Part model, mm, in its own coordinate system. A direction names the side the tool comes from. Give positions to 0.01 mm unless a question says otherwise; leave off trailing zeros. Order: outer loops, then holes, each group sorted by start corner. A loop starts at its lowest first (then second) coordinate and runs counter-clockwise, first axis right, second up.
from build123d import *

# Parameters (mm, degrees)
BOSS_EXTRUDE1_DEPTH = 3
CUT_EXTRUDE1_DEPTH  = 54.310411741


with BuildPart() as part:
    # Sketch1 → Boss-Extrude1 (new body)
    with BuildSketch(Plane.XY):
        Polygon((0, 0), (0, 45), (5, 45), (5, 48), (15, 48), (15, 45), (23, 45), (23, 27.5), (20, 27.5), (20, 17.5), (23, 17.5), (23, 0), (15, 0), (15, -6), (5, -6), (5, 0), align=None)
    extrude(amount=BOSS_EXTRUDE1_DEPTH)

    # Sketch2 → Cut-Extrude1 (cut, through all)
    with BuildSketch(Plane.XY.offset(3)):
        with BuildLine():
            Line((2.1, 42), (5.9, 42))
            ThreePointArc((5.9, 42), (5.970710678, 41.970710678), (6, 41.9))
            Line((6, 41.9), (6, 39.4))
            ThreePointArc((6, 39.4), (5.970710678, 39.329289322), (5.9, 39.3))
            Line((5.9, 39.3), (2.1, 39.3))
            ThreePointArc((2.1, 39.3), (2.029289322, 39.329289322), (2, 39.4))
            Line((2, 39.4), (2, 41.9))
            ThreePointArc((2, 41.9), (2.029289322, 41.970710678), (2.1, 42))
        make_face()
        with BuildLine():
            Line((8.1, 42), (11.9, 42))
            ThreePointArc((11.9, 42), (11.970710678, 41.970710678), (12, 41.9))
            Line((12, 41.9), (12, 39.4))
            ThreePointArc((12, 39.4), (11.970710678, 39.329289322), (11.9, 39.3))
            Line((11.9, 39.3), (8.1, 39.3))
            ThreePointArc((8.1, 39.3), (8.029289322, 39.329289322), (8, 39.4))
            Line((8, 39.4), (8, 41.9))
            ThreePointArc((8, 41.9), (8.029289322, 41.970710678), (8.1, 42))
        make_face()
        with BuildLine():
            Line((14.1, 42), (17.9, 42))
            ThreePointArc((17.9, 42), (17.970710678, 41.970710678), (18, 41.9))
            Line((18, 41.9), (18, 39.4))
            ThreePointArc((18, 39.4), (17.970710678, 39.329289322), (17.9, 39.3))
            Line((17.9, 39.3), (14.1, 39.3))
            ThreePointArc((14.1, 39.3), (14.029289322, 39.329289322), (14, 39.4))
            Line((14, 39.4), (14, 41.9))
            ThreePointArc((14, 41.9), (14.029289322, 41.970710678), (14.1, 42))
        make_face()
        with BuildLine():
            Line((8.1, 37), (11.9, 37))
            ThreePointArc((11.9, 37), (11.970710678, 36.970710678), (12, 36.9))
            Line((12, 36.9), (12, 34.4))
            ThreePointArc((12, 34.4), (11.970710678, 34.329289322), (11.9, 34.3))
            Line((11.9, 34.3), (8.1, 34.3))
            ThreePointArc((8.1, 34.3), (8.029289322, 34.329289322), (8, 34.4))
            Line((8, 34.4), (8, 36.9))
            ThreePointArc((8, 36.9), (8.029289322, 36.970710678), (8.1, 37))
        make_face()
        with BuildLine():
            Line((14.1, 37), (17.9, 37))
            ThreePointArc((17.9, 37), (17.970710678, 36.970710678), (18, 36.9))
            Line((18, 36.9), (18, 34.4))
            ThreePointArc((18, 34.4), (17.970710678, 34.329289322), (17.9, 34.3))
            Line((17.9, 34.3), (14.1, 34.3))
            ThreePointArc((14.1, 34.3), (14.029289322, 34.329289322), (14, 34.4))
            Line((14, 34.4), (14, 36.9))
            ThreePointArc((14, 36.9), (14.029289322, 36.970710678), (14.1, 37))
        make_face()
        with BuildLine():
            Line((8.1, 32), (11.9, 32))
            ThreePointArc((11.9, 32), (11.970710678, 31.970710678), (12, 31.9))
            Line((12, 31.9), (12, 29.4))
            ThreePointArc((12, 29.4), (11.970710678, 29.329289322), (11.9, 29.3))
            Line((11.9, 29.3), (8.1, 29.3))
            ThreePointArc((8.1, 29.3), (8.029289322, 29.329289322), (8, 29.4))
            Line((8, 29.4), (8, 31.9))
            ThreePointArc((8, 31.9), (8.029289322, 31.970710678), (8.1, 32))
        make_face()
        with BuildLine():
            Line((14.1, 32), (17.9, 32))
            ThreePointArc((17.9, 32), (17.970710678, 31.970710678), (18, 31.9))
            Line((18, 31.9), (18, 29.4))
            ThreePointArc((18, 29.4), (17.970710678, 29.329289322), (17.9, 29.3))
            Line((17.9, 29.3), (14.1, 29.3))
            ThreePointArc((14.1, 29.3), (14.029289322, 29.329289322), (14, 29.4))
            Line((14, 29.4), (14, 31.9))
            ThreePointArc((14, 31.9), (14.029289322, 31.970710678), (14.1, 32))
        make_face()
        with BuildLine():
            Line((2.1, 37), (5.9, 37))
            ThreePointArc((5.9, 37), (5.970710678, 36.970710678), (6, 36.9))
            Line((6, 36.9), (6, 34.4))
            ThreePointArc((6, 34.4), (5.970710678, 34.329289322), (5.9, 34.3))
            Line((5.9, 34.3), (2.1, 34.3))
            ThreePointArc((2.1, 34.3), (2.029289322, 34.329289322), (2, 34.4))
            Line((2, 34.4), (2, 36.9))
            ThreePointArc((2, 36.9), (2.029289322, 36.970710678), (2.1, 37))
        make_face()
        with BuildLine():
            Line((2.1, 32), (5.9, 32))
            ThreePointArc((5.9, 32), (5.970710678, 31.970710678), (6, 31.9))
            Line((6, 31.9), (6, 29.4))
            ThreePointArc((6, 29.4), (5.970710678, 29.329289322), (5.9, 29.3))
            Line((5.9, 29.3), (2.1, 29.3))
            ThreePointArc((2.1, 29.3), (2.029289322, 29.329289322), (2, 29.4))
            Line((2, 29.4), (2, 31.9))
            ThreePointArc((2, 31.9), (2.029289322, 31.970710678), (2.1, 32))
        make_face()
    extrude(amount=-CUT_EXTRUDE1_DEPTH, mode=Mode.SUBTRACT)


solid = part.part
Item 1: Pull direction Y, two halves, no side cores. Call faces 1 (the face through (23, 36, 1)), 2 (the face through (14, 31, 2)), 3 (the face through (19, 45, 1)): released by +Y, released by -Y, zero draft, split by the parting line, or undercut.
Item 2: Drill centre lines: probe 1 along Y at (x, z) = (17.5, 2.65); probe 2 along Y at (x, z) = (9.5, 0.3); probe 3 along Y at (x, z) = (21.25, 0.55). Where is each one in solid material? Low to high.
Item 3: Band-saw the part on D-D on y = 23.5. List the corners of the cut face in (x, z).
Item 4: Band-saw the part on A-A on x = 4.5. List the corners of the cut face in (y, z), plus the area to 3 significant figures.
Item 5: Band-saw the part on B-B on x = 9. List the corners of the cut face in (y, z).
Item 6: Band-saw the part on C-C on z = 1.4. Give the number of separate pieces and of enclosed holes in the cut face, plus the area to 3 significant figures.
Item 7: Drop flat-ended pins along their axis: P1, Ø1.5, axis at y = -4, z = 2, coming from the -X side; P2, Ø1.5, axis at x = 1.5, z = 1, coming from the +Y side; P3, Ø0.9, axis at x = 16.5, z = 1, coming from the -Y side. Give the stop position or say it passes through.
Item 8: Which spindle directions (+Z, -Z, +X, -X, +Y, -Y) get a long thin tool onto all of the face, cutting with end or side? Do faces 4 (the face through (3, 0, 1)), 5 (the face through (12, 21, 3)), 6 (the face through (10, 39.3, 2)). Say none if no direction does.
Working result:
1. face 1: zero draft
1. face 2: undercut
1. face 3: released by +Y
2. probe 1: y = 0 to 29.3, 32 to 34.3, 37 to 39.3, 42 to 45
2. probe 2: y = -6 to 29.3, 32 to 34.3, 37 to 39.3, 42 to 48
2. probe 3: y = 0 to 17.5, 27.5 to 45
3. outline: (0, 0) - (20, 0) - (20, 3) - (0, 3) - close
4. outline: (0, 0) - (29.3, 0) - (29.3, 3) - (0, 3) - close; (32, 0) - (34.3, 0) - (34.3, 3) - (32, 3) - close; (37, 0) - (39.3, 0) - (39.3, 3) - (37, 3) - close; (42, 0) - (45, 0) - (45, 3) - (42, 3) - close
4. area: 111 mm2
5. outline: (-6, 0) - (29.3, 0) - (29.3, 3) - (-6, 3) - close; (32, 0) - (34.3, 0) - (34.3, 3) - (32, 3) - close; (37, 0) - (39.3, 0) - (39.3, 3) - (37, 3) - close; (42, 0) - (48, 0) - (48, 3) - (42, 3) - close
6. separate pieces: 1
6. enclosed holes: 9
6. area: 998 mm2
7. P1: stops at x = 5
7. P2: stops at y = 45
7. P3: stops at y = 0
8. face 4: +Z, -Z, -X, -Y
8. face 5: +Z, +X, -X, +Y, -Y
8. face 6: +Z, -Z
